from build123d import *

# Parameters (mm, degrees)
EXTRUDE_1_DEPTH     = 3
EXTRUDE_2_DEPTH     = 6
CUT_EXTRUDE_1_DEPTH = 4
CHAMFER_1_SIZE      = 1


with BuildPart() as part:
    # Эскиз1 → Бобышка-Вытянуть1 (new body)
    with BuildSketch(Plane.XY):
        with BuildLine():
            Line((-6, 5), (6, 5))
            ThreePointArc((6, 5), (11, 0), (6, -5))
            Line((6, -5), (-6, -5))
            ThreePointArc((-6, -5), (-11, 0), (-6, 5))
        make_face()
    extrude(amount=EXTRUDE_1_DEPTH)

    # Эскиз2 → Бобышка-Вытянуть2 (add)
    with BuildSketch(Plane.XY.offset(3)):
        with BuildLine():
            Line((-2.5, 3.5), (2.5, 3.5))
            ThreePointArc((2.5, 3.5), (6, 0), (2.5, -3.5))
            Line((2.5, -3.5), (-2.5, -3.5))
            ThreePointArc((-2.5, -3.5), (-6, 0), (-2.5, 3.5))
        make_face()
    extrude(amount=EXTRUDE_2_DEPTH)

    # Эскиз3 → Вырез-Вытянуть1 (cut)
    with BuildSketch(Plane(origin=(0, 0, 0), x_dir=(-1, 0, 0), z_dir=(0, 0, -1))):
        with BuildLine():
            Line((0.75, -2), (-0.75, -2))
            ThreePointArc((-0.75, -2), (-2.75, 0), (-0.75, 2))
            Line((-0.75, 2), (0.75, 2))
            ThreePointArc((0.75, 2), (2.75, 0), (0.75, -2))
        make_face()
    extrude(amount=-CUT_EXTRUDE_1_DEPTH, mode=Mode.SUBTRACT)

    # Фаска1
    chamfer_1_edges = [part.edges().sort_by_distance(p)[0] for p in [
        (-6, 0, 9),
        (0, -3.5, 9),
        (6, 0, 9),
        (0, 3.5, 9),
    ]]
    chamfer(chamfer_1_edges, length=CHAMFER_1_SIZE)


solid = part.part
Source: CAD feature listing. Evaluate the final solid. Frame: model axes, mm. A direction names the side the tool comes from. Coordinates: 2 decimals unless noted, no trailing zeros. Loops run counter-clockwise (first coordinate to the right, second up) from the corner with the lowest first, then second, coordinate; pieces in that order, holes last. Notation, with made-up numbers: (-39.75, 55.5) -> (5.25, 55.5) arc R20 ccw to (5.25, 73.5) -> close; hole circle Ø1 at (7, -34). An arc over 180 degrees is marked (long way). Answer in a Markdown table with one row per item. Add a question column.
Q1. Reachability of faces 1 (the face through (6, 0, 5)), 2 (the face through (0, -3.5, 5)), 3 (the face through (0, 3.5, 5)), 4 (the face through (2.75, -0.04, 1.97)), 5 (the face through (0, -4, 3)) from +Z, -Z, +X, -X, +Y, -Y: full face, straight path, thin tool, end or side. Return the list, or none.
Q2. Pull-direction query (Y, two-part tool) for faces 6 (the face through (0, 5, 1)), 7 (the face through (-2.75, 0.04, 1.97)), 8 (the face through (-5.2, -0.1, 8.8)); classes: pulls with the +Y half, pulls with the -Y half, needs draft (parallel to the pull), parting line crosses it, or undercut.
Q3. Section A-A on x = 0.25. Return the cut outline in (y, z).
Q4. Section C-C on z = 5.75. Return the cut outline in (x, y).
Q5. Section D-D on x = -8. Return the cut outline in (y, z), and give its area (3 significant figures).
Q6. Contact query for flat-ended pins moving along their axis: pin 1 Ø2 at (x, y) = (-8.5, -4) entering from +Z; pin 2 Ø4 at (x, z) = (0.5, 4.5) entering from +Y; pin 3 Ø5 at (x, y) = (-7.5, -2) entering from +Z; pin 4 Ø3 at (x, z) = (4.5, 7) entering from +Y. Output: stop coordinate, or through.
Q7. Ray query, line 1 along Z through (x, y) = (6.25, -4.5); line 2 along X through (y, z) = (1.5, 3.75); line 3 along X through (y, z) = (1.25, 2). Return the intervals inside material, ascending.
Q8. Section B-B on y = 0. Return the cut outline in (x, z).
Computed values:
| question | item | result |
|---|---|---|
| 1 | face 1 | +Z, +X |
| 1 | face 2 | +Z, +X, -X, -Y |
| 1 | face 3 | +Z, +X, -X, +Y |
| 1 | face 4 | -Z |
| 1 | face 5 | +Z |
| 2 | face 6 | pulls with the +Y half |
| 2 | face 7 | undercut |
| 2 | face 8 | parting line crosses it |
| 3 | outline | (-5, 0) -> (-2, 0) -> (-2, 4) -> (2, 4) -> (2, 0) -> (5, 0) -> (5, 3) -> (3.5, 3) -> (3.5, 8) -> (2.5, 9) -> (-2.5, 9) -> (-3.5, 8) -> (-3.5, 3) -> (-5, 3) -> close |
| 4 | outline | (-2.5, -3.5) -> (2.5, -3.5) arc R3.5 ccw to (2.5, 3.5) -> (-2.5, 3.5) arc R3.5 ccw to start |
| 5 | outline | (-4.58, 0) -> (4.58, 0) -> (4.58, 3) -> (-4.58, 3) -> close |
| 5 | area | 27.5 mm^2 |
| 6 | pin 1 | stops at z = 3 |
| 6 | pin 2 | stops at y = 5 |
| 6 | pin 3 | stops at z = 8.61 |
| 6 | pin 4 | stops at y = 3.46 |
| 7 | line 1 | z = 0 to 3 |
| 7 | line 2 | x = -5.66 to -2.07, 2.07 to 5.66 |
| 7 | line 3 | x = -10.84 to -2.31, 2.31 to 10.84 |
| 8 | outline | (-11, 0) -> (-2.75, 0) -> (-2.75, 4) -> (2.75, 4) -> (2.75, 0) -> (11, 0) -> (11, 3) -> (6, 3) -> (6, 8) -> (5, 9) -> (-5, 9) -> (-6, 8) -> (-6, 3) -> (-11, 3) -> close |
